For this review, take the finished solid that the model builds, in its own axes (mm). Face numbers are marked on the shaded views. A direction names the side the tool comes from. Coordinates: 2 decimals unless noted, no trailing zeros. Order: outer loops, then holes, each group sorted by start corner. A loop starts at its lowest first (then second) coordinate and runs counter-clockwise, first axis right, second up.
from build123d import *

# Parameters (mm, degrees)
SKETCH1_R               = 4
SKETCH1_W               = 10
SKETCH1_H               = 50
BOSS_EXTRUDE2_DEPTH     = 20
CUT_EXTRUDE1_DEPTH      = 129.597239473
CUT_EXTRUDE1_DEPTH_BACK = 129.597239473
SKETCH4_W               = 85
SKETCH4_H               = 25
SKETCH5_W               = 25
SKETCH5_H               = 25
BOSS_EXTRUDE4_DEPTH     = 10
HOLE1_D                 = 10
HOLE1_DEPTH             = 20
HOLE1_CBORE_D           = 24
HOLE1_CBORE_DEPTH       = 3


with BuildPart() as part:
    # Sketch1 → Boss-Extrude2 (new, symmetric)
    with BuildSketch(Plane(origin=(0, 0, 0), x_dir=(1, 0, 0), z_dir=(0, 1, 0))):
        with BuildLine():
            Line((74.989948747, 70.199605335), (27.241006815, 41.300394665))
            ThreePointArc((27.241006815, 41.300394665), (25, 40.331192469), (22.580955562, 40))
            Line((22.580955562, 40), (0, 40))
            Line((0, 40), (0, -40))
            Line((0, -40), (22.580955562, -40))
            ThreePointArc((22.580955562, -40), (25, -40.331192469), (27.241006815, -41.300394665))
            Line((27.241006815, -41.300394665), (74.989948747, -70.199605335))
            ThreePointArc((74.989948747, -70.199605335), (81.12845593, -71.377734399), (86.553849817, -68.273807903))
            Line((86.553849817, -68.273807903), (102.903849817, -48.723807903))
            ThreePointArc((102.903849817, -48.723807903), (104.459747288, -46.02126616), (105, -42.95))
            Line((105, -42.95), (105, 42.95))
            ThreePointArc((105, 42.95), (104.459747288, 46.02126616), (102.903849817, 48.723807903))
            Line((102.903849817, 48.723807903), (86.553849817, 68.273807903))
            ThreePointArc((86.553849817, 68.273807903), (81.12845593, 71.377734399), (74.989948747, 70.199605335))
        make_face()
        with Locations(Location((79.65, 62.5, 0), (0, 0, 270))):
            Circle(SKETCH1_R, mode=Mode.SUBTRACT)
        with Locations(Location((96, 42.95, 0), (0, 0, 270))):
            Circle(SKETCH1_R, mode=Mode.SUBTRACT)
        with Locations(Location((96, -42.95, 0), (0, 0, 270))):
            Circle(SKETCH1_R, mode=Mode.SUBTRACT)
        with Locations(Location((79.65, -62.5, 0), (0, 0, 270))):
            Circle(SKETCH1_R, mode=Mode.SUBTRACT)
        Polygon((30.85, -31.795763765), (30.85, 31.795763765), (72.509340505, 57.009349846), (85, 42.074035282), (85, -42.074035282), (72.509340505, -57.009349846), align=None, mode=Mode.SUBTRACT)
        with Locations((9, 0)):
            Rectangle(SKETCH1_W, SKETCH1_H, mode=Mode.SUBTRACT)
    extrude(amount=BOSS_EXTRUDE2_DEPTH, both=True)

    # Sketch4 → Cut-Extrude1 (cut, two sides: drawn at the far end of the back side and taken through both)
    with BuildSketch(Plane.XY.offset(-CUT_EXTRUDE1_DEPTH_BACK)):
        with Locations((62.5, 0)):
            Rectangle(SKETCH4_W, SKETCH4_H)
    extrude(amount=CUT_EXTRUDE1_DEPTH + CUT_EXTRUDE1_DEPTH_BACK, mode=Mode.SUBTRACT)

    # Sketch5 → Boss-Extrude4 (add)
    with BuildSketch(Plane(origin=(105, 0, 0), x_dir=(0, 0, -1), z_dir=(1, 0, 0))):
        Rectangle(SKETCH5_W, SKETCH5_H)
    extrude(amount=-BOSS_EXTRUDE4_DEPTH)

    # Hole1
    with Locations(Plane.ZY):
        with Locations((0, 0)):
            CounterBoreHole(HOLE1_D / 2, HOLE1_CBORE_D / 2, HOLE1_CBORE_DEPTH, depth=HOLE1_DEPTH)


solid = part.part
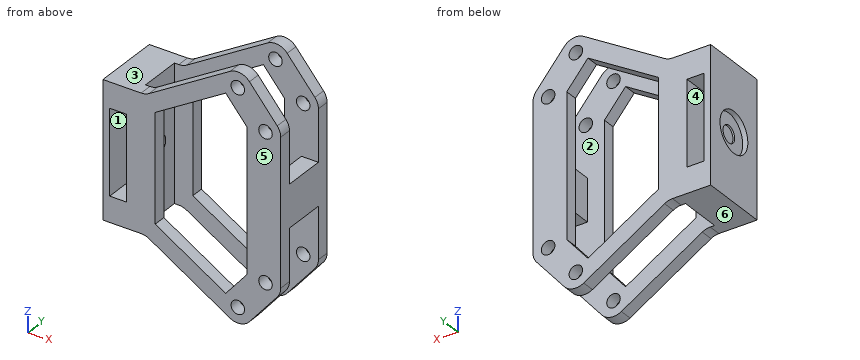
1. To check wall thickness, follow L1, parallel to Z at x = 96, y = -16.75; L2, parallel to X at y = 7.5, z = 7.5; L3, parallel to X at y = 15, z = 45. State the ranges of each line that lie inside material, in increasing order.
Answer below:
L1: z = -56.98 to -46.95, -38.95 to 38.95, 46.95 to 56.98
L2: x = 3 to 4, 14 to 20, 95 to 105
L3: x = 33.35 to 52.67, 82.55 to 92.57, 99.43 to 104.76
2. Machinability: for the marked faces 4, 5 and 6, which of the approach directions +Z, -Z, +X, -X, +Y, -Y give a long, thin tool a straight path to every point of the face, cutting with its end or side? Answer none if there is none.
Answer below:
face 4: +Y, -Y
face 5: +Z, -Z, +X, -X, -Y
face 6: -Z, -X, +Y, -Y
3. The part is to be moulded in two halves that separate along Z. For the marked faces 1, 2 and 3, say which applies: +Z half, -Z half, draft (parallel to the pull), parting line (faces both ways), or undercut.
Answer below:
face 1: undercut
face 2: draft
face 3: +Z half
4. Take a section at B-B, the plane z = -23.5. Give the boundary of the cut face in (x, y).
Answer below:
outline: (0, -20) - (4, -20) - (4, 20) - (0, 20) - close; (14, -20) - (30.85, -20) - (30.85, -12.5) - (20, -12.5) - (20, 12.5) - (30.85, 12.5) - (30.85, 20) - (14, 20) - close; (85, -20) - (105, -20) - (105, -12.5) - (85, -12.5) - close; (85, 12.5) - (105, 12.5) - (105, 20) - (85, 20) - close
5. Take a section at A-A, the plane x = 12.5. Give the boundary of the cut face in (y, z).
Answer below:
outline: (-20, -40) - (20, -40) - (20, -25) - (-20, -25) - close; (-20, 25) - (20, 25) - (20, 40) - (-20, 40) - close
6. Take a section at C-C, the plane z = 0. Give the number of separate pieces and of enclosed holes in the cut face, plus the area to 3 significant figures.
Answer below:
separate pieces: 5
enclosed holes: 0
area: 971 mm2
7. Take a section at D-D, the plane y = 14. Give the boundary of the cut face in (x, z).
Answer below:
outline: (0, -40) - (22.58, -40) arc R9 cw to (27.24, -41.3) - (74.99, -70.2) arc R9 ccw to (86.55, -68.27) - (102.9, -48.72) arc R9 ccw to (105, -42.95) - (105, 42.95) arc R9 ccw to (102.9, 48.72) - (86.55, 68.27) arc R9 ccw to (74.99, 70.2) - (27.24, 41.3) arc R9 cw to (22.58, 40) - (0, 40) - close; hole (4, -25) - (14, -25) - (14, 25) - (4, 25) - close; hole (30.85, -31.8) - (72.51, -57.01) - (85, -42.07) - (85, 42.07) - (72.51, 57.01) - (30.85, 31.8) - close; hole circle Ø8 at (79.65, -62.5); hole circle Ø8 at (79.65, 62.5); hole circle Ø8 at (96, -42.95); hole circle Ø8 at (96, 42.95)
8. Clearance check with flat-ended pins moving along their axes: pin 1 Ø2 at (y, z) = (3, 24.5) entering from +X; pin 2 Ø10 at (x, y) = (90, 15) entering from -Z; pin 3 Ø3 at (x, y) = (12, -9) entering from -Z; pin 4 Ø6.5 at (x, z) = (79.65, 62.5) entering from -Y. State where each tip first meets the part, or that it passes through.
Answer below:
pin 1: stops at x = 20
pin 2: stops at z = -69.74
pin 3: stops at z = -40
pin 4: passes through
